Model file for the job. Use its own axes, mm. A direction names the side the tool comes from. Round coordinates to 2 decimals unless told otherwise and drop trailing zeros. Loops run counter-clockwise (first coordinate to the right, second up) from the corner with the lowest first, then second, coordinate; pieces in that order, holes last.
from build123d import *

# Parameters (mm, degrees)
SKETCH3_W           = 110
SKETCH3_H           = 133
BOSS_EXTRUDE1_DEPTH = 5
SKETCH4_W           = 110
SKETCH4_H           = 133
SKETCH4_W_2         = 102
SKETCH4_H_2         = 125
BOSS_EXTRUDE2_DEPTH = 245
CUT_EXTRUDE1_DEPTH  = 282.108964638
SKETCH6_W           = 62.5
SKETCH6_H           = 25
BOSS_EXTRUDE3_DEPTH = 20
SKETCH7_R           = 2.75
CUT_EXTRUDE2_DEPTH  = 20
SKETCH8_W           = 12.5
SKETCH8_H           = 20
BOSS_EXTRUDE4_DEPTH = 20
SKETCH9_R           = 3.25
CUT_EXTRUDE3_DEPTH  = 20
SKETCH10_W          = 20
SKETCH10_H          = 2.25
CUT_EXTRUDE4_DEPTH  = 12.6
SKETCH12_W          = 20
SKETCH12_H          = 2.25
CUT_EXTRUDE5_DEPTH  = 12.6
FILLET1_R           = 2
FILLET2_R           = 2
SKETCH13_W          = 1
SKETCH13_H          = 5.289798983
CUT_EXTRUDE6_DEPTH  = 20
SKETCH14_R          = 1.375
CUT_EXTRUDE7_DEPTH  = 20
SKETCH15_R          = 1.375
CUT_EXTRUDE8_DEPTH  = 20
SKETCH16_R          = 3.75
CUT_EXTRUDE9_DEPTH  = 3
CUT_EXTRUDE10_START = -3
SKETCH17_R          = 3.75
CUT_EXTRUDE10_DEPTH = 3
SKETCH18_R          = 3.41
CUT_EXTRUDE11_DEPTH = 5
SKETCH19_R          = 3.41
CUT_EXTRUDE12_DEPTH = 5
CUT_EXTRUDE13_DEPTH = 5
SKETCH21_R          = 7.5
CUT_EXTRUDE14_DEPTH = 5
SKETCH22_R          = 3.41
CUT_EXTRUDE15_DEPTH = 5
CUT_EXTRUDE16_DEPTH = 5


with BuildPart() as part:
    # Sketch3 → Boss-Extrude1 (new body)
    with BuildSketch(Plane(origin=(0, 0, 0), x_dir=(1, 0, 0), z_dir=(0, 1, 0))):
        Rectangle(SKETCH3_W, SKETCH3_H)
    extrude(amount=BOSS_EXTRUDE1_DEPTH)

    # Sketch4 → Boss-Extrude2 (add)
    with BuildSketch(Plane(origin=(0, 5, 0), x_dir=(1, 0, 0), z_dir=(0, 1, 0))):
        Rectangle(SKETCH4_W, SKETCH4_H)
        Rectangle(SKETCH4_W_2, SKETCH4_H_2, mode=Mode.SUBTRACT)
    extrude(amount=BOSS_EXTRUDE2_DEPTH)

    # Sketch5 → Cut-Extrude1 (cut, through all)
    with BuildSketch(Plane.ZY.offset(55)):
        Polygon((-13.5, 250), (-13.5, 150), (-3.5, 150), (62.5, 38.76), (62.5, 27.9), (66.5, 27.9), (66.5, 250), align=None)
    extrude(amount=-CUT_EXTRUDE1_DEPTH, mode=Mode.SUBTRACT)

    # Sketch6 → Boss-Extrude3 (add)
    with BuildSketch(Plane(origin=(0, 5, 0), x_dir=(1, 0, 0), z_dir=(0, 1, 0))):
        with Locations((0.25, 50)):
            Rectangle(SKETCH6_W, SKETCH6_H)
    extrude(amount=BOSS_EXTRUDE3_DEPTH)

    # Sketch7 → Cut-Extrude2 (cut)
    with BuildSketch(Plane(origin=(0, 25, 0), x_dir=(1, 0, 0), z_dir=(0, 1, 0))):
        with Locations(Location((0.25, 45, 0), (0, 0, 270))):
            Circle(SKETCH7_R)
    extrude(amount=-CUT_EXTRUDE2_DEPTH, mode=Mode.SUBTRACT)

    # Sketch8 → Boss-Extrude4 (add)
    with BuildSketch(Plane(origin=(0, 5, 0), x_dir=(1, 0, 0), z_dir=(0, 1, 0))):
        with Locations((-24.75, 27.5)):
            Rectangle(SKETCH8_W, SKETCH8_H)
        with Locations((25.25, 27.5)):
            Rectangle(SKETCH8_W, SKETCH8_H)
    extrude(amount=BOSS_EXTRUDE4_DEPTH)

    # Sketch9 → Cut-Extrude3 (cut)
    with BuildSketch(Plane(origin=(0, 25, 0), x_dir=(1, 0, 0), z_dir=(0, 1, 0))):
        with Locations(Location((-24.75, 25, 0), (0, 0, 270))):
            Circle(SKETCH9_R)
        with Locations(Location((25.25, 25, 0), (0, 0, 270))):
            Circle(SKETCH9_R)
    extrude(amount=-CUT_EXTRUDE3_DEPTH, mode=Mode.SUBTRACT)

    # Sketch10 → Cut-Extrude4 (cut)
    with BuildSketch(Plane(origin=(-18.5, 0, 0), x_dir=(0, 0, -1), z_dir=(1, 0, 0))):
        with Locations((27.5, 6.125)):
            Rectangle(SKETCH10_W, SKETCH10_H)
    extrude(amount=-CUT_EXTRUDE4_DEPTH, mode=Mode.SUBTRACT)

    # Sketch12 → Cut-Extrude5 (cut)
    with BuildSketch(Plane.ZY.offset(-19)):
        with Locations((-27.5, 6.125)):
            Rectangle(SKETCH12_W, SKETCH12_H)
    extrude(amount=-CUT_EXTRUDE5_DEPTH, mode=Mode.SUBTRACT)

    # Fillet1
    fillet1_edges = [part.edges().sort_by_distance(p)[0] for p in [
        (31.5, 16.125, -17.5),
    ]]
    fillet(fillet1_edges, radius=FILLET1_R)

    # Fillet2
    fillet2_edges = [part.edges().sort_by_distance(p)[0] for p in [
        (-31, 16.125, -17.5),
    ]]
    fillet(fillet2_edges, radius=FILLET2_R)

    # Sketch13 → Cut-Extrude6 (cut)
    with BuildSketch(Plane(origin=(0, 25, 0), x_dir=(1, 0, 0), z_dir=(0, 1, 0))):
        with Locations((25.25, 20.144899491)):
            Rectangle(SKETCH13_W, SKETCH13_H)
        with Locations((-24.75, 20.144899491)):
            Rectangle(SKETCH13_W, SKETCH13_H)
    extrude(amount=-CUT_EXTRUDE6_DEPTH, mode=Mode.SUBTRACT)

    # Sketch14 → Cut-Extrude7 (cut)
    with BuildSketch(Plane(origin=(-18.5, 0, 0), x_dir=(0, 0, -1), z_dir=(1, 0, 0))):
        with Locations((20, 20)):
            Circle(SKETCH14_R)
        with Locations((20, 10)):
            Circle(SKETCH14_R)
    extrude(amount=-CUT_EXTRUDE7_DEPTH, mode=Mode.SUBTRACT)

    # Sketch15 → Cut-Extrude8 (cut)
    with BuildSketch(Plane.ZY.offset(-19)):
        with Locations((-19.75, 20)):
            Circle(SKETCH15_R)
        with Locations((-19.75, 10)):
            Circle(SKETCH15_R)
    extrude(amount=-CUT_EXTRUDE8_DEPTH, mode=Mode.SUBTRACT)

    # Sketch16 → Cut-Extrude9 (cut)
    with BuildSketch(Plane.ZY.offset(31)):
        with Locations((-20, 20)):
            Circle(SKETCH16_R)
        with Locations((-20, 10)):
            Circle(SKETCH16_R)
    extrude(amount=-CUT_EXTRUDE9_DEPTH, mode=Mode.SUBTRACT)

    # Sketch17 → Cut-Extrude10 (cut)
    with BuildSketch(Plane(origin=(31.5, 0, 0), x_dir=(0, 0, -1), z_dir=(1, 0, 0)).offset(CUT_EXTRUDE10_START)):
        with Locations((20, 20)):
            Circle(SKETCH17_R)
        with Locations((20, 10)):
            Circle(SKETCH17_R)
    extrude(amount=CUT_EXTRUDE10_DEPTH, mode=Mode.SUBTRACT)

    # Sketch18 → Cut-Extrude11 (cut)
    with BuildSketch(Plane.XY.offset(66.5)):
        with Locations((-40, 17.9)):
            Circle(SKETCH18_R)
        with Locations((40, 17.9)):
            Circle(SKETCH18_R)
    extrude(amount=-CUT_EXTRUDE11_DEPTH, mode=Mode.SUBTRACT)

    # Sketch19 → Cut-Extrude12 (cut)
    with BuildSketch(Plane.ZY.offset(55)):
        with Locations((-46.5, 120)):
            Circle(SKETCH19_R)
        with Locations((-46.5, 20)):
            Circle(SKETCH19_R)
        with Locations((46.5, 20)):
            Circle(SKETCH19_R)
    extrude(amount=-CUT_EXTRUDE12_DEPTH, mode=Mode.SUBTRACT)

    # Sketch20 → Cut-Extrude13 (cut)
    with BuildSketch(Plane.ZY.offset(55)):
        with BuildLine():
            Line((3.133380894, 138.819738021), (-6.861130368, 133.308120044))
            ThreePointArc((-6.861130368, 133.308120044), (-15.692800866, 135.862800883), (-13.135528331, 144.693721286))
            Line((-13.135528331, 144.693721286), (-3.5, 150))
            Line((-3.5, 150), (3.133380894, 138.819738021))
        make_face()
    extrude(amount=-CUT_EXTRUDE13_DEPTH, mode=Mode.SUBTRACT)

    # Sketch21 → Cut-Extrude14 (cut)
    with BuildSketch(Plane(origin=(55, 0, 0), x_dir=(0, 0, -1), z_dir=(1, 0, 0))):
        with Locations((-16.5, 15)):
            Circle(SKETCH21_R)
    extrude(amount=-CUT_EXTRUDE14_DEPTH, mode=Mode.SUBTRACT)

    # Sketch22 → Cut-Extrude15 (cut)
    with BuildSketch(Plane(origin=(55, 0, 0), x_dir=(0, 0, -1), z_dir=(1, 0, 0))):
        with Locations((-26.5, 35)):
            Circle(SKETCH22_R)
        with Locations((23.5, 35)):
            Circle(SKETCH22_R)
    extrude(amount=-CUT_EXTRUDE15_DEPTH, mode=Mode.SUBTRACT)

    # Sketch23 → Cut-Extrude16 (cut)
    with BuildSketch(Plane(origin=(55, 0, 0), x_dir=(0, 0, -1), z_dir=(1, 0, 0))):
        with BuildLine():
            Line((36.5, 224), (36.5, 229.629285786))
            ThreePointArc((36.5, 229.629285786), (40, 238.2), (43.5, 229.629285786))
            Line((43.5, 229.629285786), (43.5, 224))
            ThreePointArc((43.5, 224), (40, 220.5), (36.5, 224))
        make_face()
        with BuildLine():
            Line((36.5, 184), (36.5, 189.629285786))
            ThreePointArc((36.5, 189.629285786), (40, 198.2), (43.5, 189.629285786))
            Line((43.5, 189.629285786), (43.5, 184))
            ThreePointArc((43.5, 184), (40, 180.5), (36.5, 184))
        make_face()
    extrude(amount=-CUT_EXTRUDE16_DEPTH, mode=Mode.SUBTRACT)


solid = part.part
Q1. Slice it at C-C on x = 10. Give the cut face in (y, z), plus the area to 3 significant figures.
Q2. Slice it at A-A on y = 233.2. Give the cut face in (x, z), plus the area to 3 significant figures.
Q3. Flat gauge pins, fed straight in: P1, Ø12, axis at x = 18, y = 112.5, coming from the +Z side; P2, Ø1.5, axis at x = -13, z = 21, coming from the -Y side; P3, Ø6, axis at x = -35.5, z = 47, coming from the +Y side; P4, Ø2, axis at x = -20.5, z = 64.5, coming from the +Y side. Where does each tip first touch, or does it go through?
Q4. Slice it at D-D on y = 92. Give the cut face in (x, z), plus the area to 3 significant figures.
Q5. Probe line 1 (X direction, y = 13, z = -45); line 2 (Y direction, x = -20, z = -20) (3 decimals); line 3 (X direction, y = 20, z = -25). List the from-to ranges inside material, lowest first.
Q6. Slice it at B-B on x = 40. Give the cut face in (y, z).
Q7. Tool access for faces 4 (the face through (36.593, 18.05, 64.528)), 5 (the face through (51, 99, -13)), 6 (the face through (52.972, 95.159, 29.038)), 7 (the face through (-29.52, 20.12, -23.75)), 8 (the face through (53.028, 238.197, -39.834)): list every direction of +Z, -Z, +X, -X, +Y, -Y with a clear straight run to the whole face (end or side of a thin tool).
Q8. Pull direction Y, two halves, no side cores. Call faces 1 (the face through (-53.028, 20.15, 43.093)), 2 (the face through (0, 25, -40)), 3 (the face through (25.386, 16.249, -28.247)): pulls with the +Y half, pulls with the -Y half, needs draft (parallel to the pull), parting line crosses it, or undercut.
Reply:
1. outline: (0, -66.5) - (250, -66.5) - (250, -62.5) - (25, -62.5) - (25, -37.5) - (5, -37.5) - (5, 62.5) - (27.9, 62.5) - (27.9, 66.5) - (0, 66.5) - close
1. area: 2,240 mm2
2. outline: (-55, -66.5) - (55, -66.5) - (55, -45) - (51, -45) - (51, -62.5) - (-51, -62.5) - (-51, -13.5) - (-55, -13.5) - close; (51, -35) - (55, -35) - (55, -13.5) - (51, -13.5) - close
2. area: 792 mm2
3. P1: stops at z = -62.5
3. P2: stops at y = 0
3. P3: stops at y = 5
3. P4: stops at y = 27.9
4. outline: (-55, -66.5) - (55, -66.5) - (55, 30.91) - (51, 30.91) - (51, -62.5) - (-51, -62.5) - (-51, 30.91) - (-55, 30.91) - close
4. area: 1,190 mm2
5. line 1: x = -55 to -51, -31 to -2.5, 3 to 31.5, 51 to 55
5. line 2: y = 0 to 5, 7.25 to 8.625, 11.375 to 18.625, 21.375 to 25
5. line 3: x = -55 to -51, -31 to -28, -21.5 to -18.5, 19 to 22, 28.5 to 31.5, 51 to 55
6. outline: (0, -66.5) - (250, -66.5) - (250, -62.5) - (5, -62.5) - (5, 62.5) - (14.49, 62.5) - (14.49, 66.5) - (0, 66.5) - close; (21.31, 62.5) - (27.9, 62.5) - (27.9, 66.5) - (21.31, 66.5) - close
7. face 4: +Z
7. face 5: +Y
7. face 6: +Z, +X, -X, +Y
7. face 7: none
7. face 8: +X
8. face 1: undercut
8. face 2: pulls with the +Y half
8. face 3: needs draft
